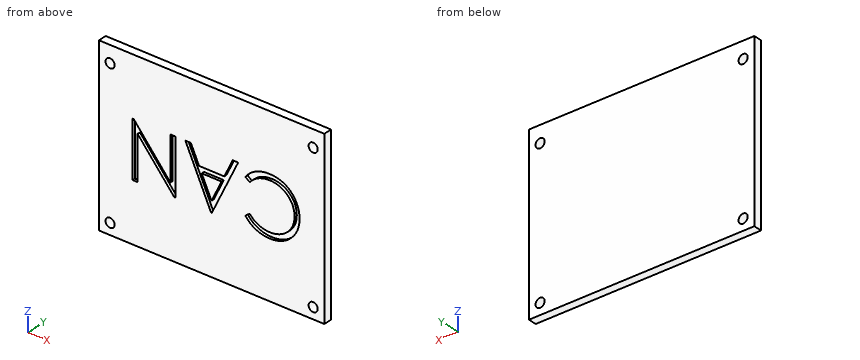
```python
from build123d import *

# Parameters (mm, degrees)
SKETCH1_W      = 81
SKETCH1_H      = 62
EXTRUDE1_DEPTH = 3
SKETCH2_R      = 1.65
EXTRUDE2_DEPTH = 3
EXTRUDE3_START = -1
EXTRUDE3_DEPTH = 1


# Read off the part's stored shape, not the designer's step: Extrude3
with BuildPart() as part:
    # Sketch1 → Extrude1 (new body)
    with BuildSketch(Plane(origin=(0, 0, 0), x_dir=(1, 0, 0), z_dir=(0, 1, 0))):
        Rectangle(SKETCH1_W, SKETCH1_H)
    extrude(amount=EXTRUDE1_DEPTH)

    # Sketch2 → Extrude2 (cut)
    with BuildSketch(Plane(origin=(0, 3, 0), x_dir=(1, 0, 0), z_dir=(0, 1, 0))):
        with Locations(Location((-36.5, 27, 0), (0, 0, 270))):
            Circle(SKETCH2_R)
        with Locations(Location((36.5, 27, 0), (0, 0, 270))):
            Circle(SKETCH2_R)
        with Locations(Location((36.5, -25, 0), (0, 0, 270))):
            Circle(SKETCH2_R)
        with Locations(Location((-36.5, -25, 0), (0, 0, 270))):
            Circle(SKETCH2_R)
    extrude(amount=-EXTRUDE2_DEPTH, mode=Mode.SUBTRACT)

    # Extrude3 outline → Extrude3 (cut)
    # profile 1 of 3: a face of its own
    with BuildSketch(Plane(origin=(0, 0, 0), x_dir=(-1, 0, 0), z_dir=(0, -1, 0)).offset(EXTRUDE3_START)):
        with BuildLine():
            add(Edge.make_bspline(
                [(-20.83620317, 10.515533954), (-20.606406188, 10.512778879), (-20.151546203, 10.507325485), (-19.478673903, 10.45414753), (-18.823574892, 10.365498351), (-18.185797852, 10.244835095), (-17.562240045, 10.095078972), (-16.95766724, 9.899991553), (-16.368531887, 9.67692566), (-15.798549554, 9.420020141), (-15.250454982, 9.131638761), (-14.724418876, 8.814978055), (-14.224619684, 8.470430595), (-13.74754055, 8.100926736), (-13.301162201, 7.698649254), (-12.872810895, 7.274662991), (-12.477033305, 6.816755425), (-12.232729334, 6.494441517), (-12.110241632, 6.332841646)],
                knots=[0, 0, 0, 0, 0.068547537, 0.135682946, 0.20121499, 0.265682235, 0.329266835, 0.392395428, 0.455069762, 0.51712685, 0.578790035, 0.639739863, 0.700191504, 0.759806243, 0.819628319, 0.879354791, 0.939511608, 1, 1, 1, 1], degree=3))
            add(Edge.make_bspline(
                [(-31.597421119, 0.118899339), (-31.588534298, 0.478644788), (-31.571050034, 1.186421499), (-31.422502632, 2.225129804), (-31.183538082, 3.220280654), (-30.84412729, 4.170016338), (-30.413810997, 5.079332225), (-29.882230346, 5.941281967), (-29.255560962, 6.761377965), (-28.538717718, 7.527176544), (-27.752618659, 8.227401416), (-26.910796866, 8.843436866), (-26.014900026, 9.356108386), (-25.074798016, 9.784657885), (-24.083451264, 10.114054818), (-23.042974869, 10.344644456), (-21.955323928, 10.488170835), (-21.213252924, 10.50631488), (-20.83620317, 10.515533954)],
                knots=[0, 0, 0, 0, 0.064557846, 0.127013532, 0.18795481, 0.248013913, 0.307747682, 0.368234515, 0.429469844, 0.492743437, 0.556257769, 0.618216786, 0.679655476, 0.741245546, 0.803415265, 0.866815462, 0.932328312, 1, 1, 1, 1], degree=3))
            add(Edge.make_bspline(
                [(-29.061363426, -7.012510918), (-29.263852818, -6.763704124), (-29.666386971, -6.26909435), (-30.181390877, -5.467460171), (-30.62223405, -4.630498978), (-30.978667883, -3.753813671), (-31.257312072, -2.839371458), (-31.450347473, -1.886711375), (-31.575785213, -0.896723134), (-31.59012972, -0.223370056), (-31.597421119, 0.118899339)],
                knots=[0, 0, 0, 0, 0.12432851, 0.247156016, 0.368779749, 0.490733862, 0.613613772, 0.738957576, 0.867310575, 1, 1, 1, 1], degree=3))
            add(Edge.make_bspline(
                [(-20.812164709, -10.510107071), (-21.027271377, -10.508609971), (-21.452618178, -10.505649641), (-22.080611044, -10.457694398), (-22.691980077, -10.39226733), (-23.28497794, -10.293752296), (-23.862840654, -10.177498924), (-24.420329708, -10.021663172), (-24.96293091, -9.847096505), (-25.488464286, -9.641925153), (-25.997376856, -9.41040411), (-26.488027207, -9.148738059), (-26.960189678, -8.859127403), (-27.418506368, -8.547955915), (-27.856206846, -8.205228476), (-28.277084134, -7.83570485), (-28.683498284, -7.440630503), (-28.934942198, -7.155745627), (-29.061363426, -7.012510918)],
                knots=[0, 0, 0, 0, 0.069662801, 0.137749562, 0.203916744, 0.268779862, 0.332413706, 0.39475354, 0.456180032, 0.516995649, 0.577395938, 0.637198344, 0.696999184, 0.756756194, 0.816553905, 0.876947997, 0.938131788, 1, 1, 1, 1], degree=3))
            add(Edge.make_bspline(
                [(-12.110241632, -6.315395533), (-12.236630831, -6.478472401), (-12.488803832, -6.803845008), (-12.897135358, -7.262540493), (-13.327291343, -7.693992124), (-13.782466829, -8.094721388), (-14.257425638, -8.472746906), (-14.760695994, -8.817328799), (-15.285661894, -9.133276709), (-15.830544631, -9.422573421), (-16.394765275, -9.679243404), (-16.977647761, -9.89897922), (-17.576679621, -10.088264303), (-18.19188824, -10.243989655), (-18.824549708, -10.365538706), (-19.472380989, -10.446793991), (-20.136780275, -10.502462073), (-20.585016968, -10.507535878), (-20.812164709, -10.510107071)],
                knots=[0, 0, 0, 0, 0.061674239, 0.123053062, 0.183475001, 0.243726501, 0.304278917, 0.364862921, 0.425946204, 0.48739123, 0.549220384, 0.611143589, 0.67352853, 0.736961457, 0.800785283, 0.866012596, 0.932100748, 1, 1, 1, 1], degree=3))
            Line((-12.110241632, -6.315395533), (-13.680754452, -5.125491687))
            add(Edge.make_bspline(
                [(-20.824183939, -8.45882502), (-20.475025716, -8.44917485), (-19.787798808, -8.430181007), (-18.779981515, -8.269271012), (-17.815205711, -8.008368624), (-16.893419503, -7.64323764), (-16.017221524, -7.168578852), (-15.185240608, -6.593162409), (-14.396774491, -5.911514794), (-13.922652878, -5.391039775), (-13.680754452, -5.125491687)],
                knots=[0, 0, 0, 0, 0.12851519, 0.252948636, 0.374754734, 0.495939754, 0.617180641, 0.740909469, 0.867811148, 1, 1, 1, 1], degree=3))
            add(Edge.make_bspline(
                [(-29.802549324, -0.01731861), (-29.795338929, -0.312926152), (-29.781182276, -0.893312351), (-29.655191796, -1.743430126), (-29.463734131, -2.557833976), (-29.176787978, -3.331433075), (-28.822964831, -4.07376655), (-28.375875623, -4.772274283), (-27.858066838, -5.437511795), (-27.262213012, -6.053757211), (-26.608465493, -6.616692784), (-25.907048855, -7.112410392), (-25.159710068, -7.525638292), (-24.374700752, -7.869500844), (-23.545980101, -8.133825002), (-22.675038373, -8.319905708), (-21.763769829, -8.441289596), (-21.141087544, -8.452910671), (-20.824183939, -8.45882502)],
                knots=[0, 0, 0, 0, 0.064323217, 0.126290104, 0.186726469, 0.246146432, 0.305575643, 0.365429386, 0.426326309, 0.488839906, 0.551724972, 0.613918596, 0.675483766, 0.737333897, 0.800229044, 0.864502298, 0.931040739, 1, 1, 1, 1], degree=3))
            add(Edge.make_bspline(
                [(-20.948382657, 8.464251903), (-21.148858653, 8.461943546), (-21.54795004, 8.457348255), (-22.140227031, 8.396724682), (-22.721444466, 8.311517768), (-23.291224273, 8.185087349), (-23.848841179, 8.025243812), (-24.397940619, 7.834241447), (-24.930572618, 7.597928076), (-25.454105408, 7.336738019), (-25.955700899, 7.041724049), (-26.430301172, 6.719933467), (-26.876175275, 6.374967202), (-27.293675916, 6.005532308), (-27.683229906, 5.613292534), (-28.042014539, 5.194067725), (-28.368788312, 4.749198162), (-28.670028455, 4.284550119), (-28.939815503, 3.801477024), (-29.165700528, 3.298190907), (-29.365729798, 2.783310318), (-29.524011185, 2.25101797), (-29.649294138, 1.705059308), (-29.735737928, 1.143969092), (-29.795672049, 0.568919494), (-29.800244489, 0.179151993), (-29.802549324, -0.01731861)],
                knots=[0, 0, 0, 0, 0.043954909, 0.087501875, 0.130462627, 0.172752021, 0.215403067, 0.25764983, 0.300152749, 0.34312149, 0.385925163, 0.427685727, 0.46881795, 0.5094918, 0.549883031, 0.589980023, 0.63040523, 0.670868626, 0.711383944, 0.751627258, 0.791775577, 0.832458919, 0.873319045, 0.914542956, 0.956923558, 1, 1, 1, 1], degree=3))
            add(Edge.make_bspline(
                [(-13.680754452, 5.13091857), (-13.7927881, 5.264438397), (-14.015344939, 5.529677916), (-14.373397525, 5.902132455), (-14.74654977, 6.251076806), (-15.134659034, 6.578173261), (-15.544711145, 6.871983351), (-15.966772852, 7.147818225), (-16.407904539, 7.395062442), (-17.017914451, 7.694850934), (-17.815902156, 8.007686106), (-18.820444093, 8.269990285), (-19.869078942, 8.436968431), (-20.584493797, 8.45505324), (-20.948382657, 8.464251903)],
                knots=[0, 0, 0, 0, 0.063163259, 0.125474941, 0.18712122, 0.248294346, 0.309294856, 0.369850066, 0.430973376, 0.49245599, 0.616147966, 0.740843698, 0.868182649, 1, 1, 1, 1], degree=3))
            Line((-13.680754452, 5.13091857), (-12.110241632, 6.332841646))
        make_face()
    # profile 2 of 3: a face of its own
    with BuildSketch(Plane(origin=(0, 0, 0), x_dir=(-1, 0, 0), z_dir=(0, -1, 0)).offset(EXTRUDE3_START)):
        Polygon((13.017963497, -9.997286559), (14.812835291, -9.997286559), (14.812835291, 5.707841646), (27.993925035, -9.997286559), (28.402578881, -9.997286559), (28.402578881, 10.002713441), (26.607707086, 10.002713441), (26.607707086, -5.738472456), (13.394566061, 10.002713441), (13.017963497, 10.002713441), align=None)
    # profile 3 of 3: a face of its own
    with BuildSketch(Plane(origin=(0, 0, 0), x_dir=(-1, 0, 0), z_dir=(0, -1, 0)).offset(EXTRUDE3_START)):
        Polygon((7.477098112, -9.997286559), (9.428219907, -9.997286559), (0.197450676, 10.002713441), (-0.05895958, 10.002713441), (-9.546139067, -9.997286559), (-7.587004452, -9.997286559), (-4.546139067, -3.587030148), (4.520367343, -3.587030148), align=None)
        Polygon((0.049213497, 6.104476262), (3.574854522, -1.535748097), (-3.572581375, -1.535748097), align=None, mode=Mode.SUBTRACT)
    extrude(amount=EXTRUDE3_DEPTH, mode=Mode.SUBTRACT)


solid = part.part
```
Verification items for the finished model (mm, model axes). Coordinates: 2 decimals unless noted, no trailing zeros. Loops run counter-clockwise (first coordinate to the right, second up) from the corner with the lowest first, then second, coordinate; pieces in that order, holes last. Notation, with made-up numbers: (-32.75, 34.25) -> (-9.75, 34.25) arc R14 ccw to (-9.75, 42.25) -> close; hole circle Ø1 at (71.25, 22). An arc over 180 degrees is marked (long way). Answer in a Markdown table with one row per item.
1) Scan lines: line 1 along X through (y, z) = (2.15, -27); line 2 along X through (y, z) = (2.2, 24); line 3 along Z through (x, y) = (-3, 0.8). Record each from-to range of solid material in increasing order. Write a range as from..to.
The answers:
| item | result |
|---|---|
| line 1 | x = -40.5..-38.15, -34.85..34.85, 38.15..40.5 |
| line 2 | x = -40.5..-37.81, -35.19..35.19, 37.81..40.5 |
| line 3 | z = -31..-3.93, 0.29..1.54, 3.59..31 |
2) Section check B-B (z = 25). Record the cut outline in (x, y), and give its area (3 significant figures).
The answers:
| item | result |
|---|---|
| outline | (-40.5, 0) -> (-38.15, 0) -> (-38.15, 3) -> (-40.5, 3) -> close; (-34.85, 0) -> (34.85, 0) -> (34.85, 3) -> (-34.85, 3) -> close; (38.15, 0) -> (40.5, 0) -> (40.5, 3) -> (38.15, 3) -> close |
| area | 223 mm2 |
3) Section check A-A (x = -36.5). Record the cut outline in (y, z).
The answers:
| item | result |
|---|---|
| outline | (0, -31) -> (3, -31) -> (3, -28.65) -> (0, -28.65) -> close; (0, -25.35) -> (3, -25.35) -> (3, 23.35) -> (0, 23.35) -> close; (0, 26.65) -> (3, 26.65) -> (3, 31) -> (0, 31) -> close |
